```python
from build123d import *

# Parameters (mm, degrees)
F0_W     = 42
F0_H     = 15
F1_DEPTH = 1.5
F2_R     = 3.5
F3_DEPTH = 0.25
F4_R     = 1.25
F5_DEPTH = 5
F6_R     = 1
F7_DEPTH = 5
F9_DEPTH = 1.2


with BuildPart() as f1:
    # F0 (on Top) → F1 (new body)
    with BuildSketch(Plane.XY):
        with Locations((-10.6229138038, 35.7527500853)):
            Rectangle(F0_W, F0_H)
        with BuildLine():
            Line((10.3770861962, 18.2527500853), (10.3770861962, 28.2527500853))
            Line((10.3770861962, 28.2527500853), (-31.6229138038, 28.2527500853))
            Line((-31.6229138038, 28.2527500853), (-31.6229138038, 21.7527500853))
            ThreePointArc((-31.6229138038, 21.7527500853), (-29.8655544909, 17.5101093982), (-25.6229138038, 15.7527500853))
            Line((-25.6229138038, 15.7527500853), (-24.5371273662, 15.7527500853))
            Line((-24.5371273662, 15.7527500853), (-23.1229138038, 15.7527500853))
            Line((-23.1229138038, 15.7527500853), (5.8770861962, 15.7527500853))
            Line((5.8770861962, 15.7527500853), (10.3770861962, 15.7527500853))
            Line((10.3770861962, 15.7527500853), (10.3770861962, 18.2527500853))
        make_face()
        Polygon((43.8770861962, 28.2527500853), (10.3770861962, 28.2527500853), (10.3770861962, 18.2527500853), (31.8770861962, 18.2527500853), (43.8770861962, 18.2527500853), align=None)
        Polygon((31.8770861962, 18.2527500853), (10.3770861962, 18.2527500853), (10.3770861962, 15.7527500853), (22.8770861962, 15.7527500853), (31.8770861962, 15.7527500853), align=None)
        Polygon((22.8770861962, 15.7527500853), (10.3770861962, 15.7527500853), (5.8770861962, 15.7527500853), (5.8770861962, -13.6921136433), align=None)
        Polygon((5.8770861962, -13.6921136433), (5.8770861962, 15.7527500853), (-23.1229138038, 15.7527500853), (-23.1229138038, 11.7527500853), (-23.1229138038, 10.6903063133), (-23.1229138038, -9.6921136433), (-23.1229138038, -13.6921136433), (-2.5732517242, -13.6921136433), (-1.1229138038, -13.6921136433), (2.8770861962, -13.6921136433), (4.2299595661, -13.6921136433), align=None)
        with BuildLine():
            Line((-24.5371273662, 15.7527500853), (-25.6229138038, 15.7527500853))
            add(Edge.make_bspline(
                [(-25.6229138038, 15.7527500853), (-25.2405945212, 15.277672559), (-25.4562471371, 14.5860834187), (-25.3729138038, 14.0027500853)],
                knots=[0, 0, 0, 0, 1.767766953, 1.767766953, 1.767766953, 1.767766953], degree=3))
            ThreePointArc((-25.3729138038, 14.0027500853), (-25.1532438897, 14.9724199994), (-24.5371273662, 15.7527500853))
        make_face()
        with BuildLine():
            Line((-23.1229138038, 11.7527500853), (-23.1229138038, 15.7527500853))
            Line((-23.1229138038, 15.7527500853), (-24.5371273662, 15.7527500853))
            ThreePointArc((-24.5371273662, 15.7527500853), (-25.1532438897, 14.9724199994), (-25.3729138038, 14.0027500853))
            ThreePointArc((-25.3729138038, 14.0027500853), (-24.934409558, 12.6682152852), (-23.7898176859, 11.8538575305))
            ThreePointArc((-23.7898176859, 11.8538575305), (-23.4601761288, 11.7781705466), (-23.1229138038, 11.7527500853))
        make_face()
        with BuildLine():
            Line((-23.1229138038, -13.6921136433), (-23.1229138038, -9.6921136433))
            ThreePointArc((-23.1229138038, -9.6921136433), (-25.1229138038, -11.6921136433), (-23.1229138038, -13.6921136433))
        make_face()
        with BuildLine():
            add(Edge.make_bspline(
                [(2.6500229876, -14.6176919133), (3.1772305838, -14.3094592572), (3.4171862062, -13.6921136433), (4.2299595661, -13.6921136433)],
                knots=[0, 0, 0, 0, 1.8310911299, 1.8310911299, 1.8310911299, 1.8310911299], degree=3))
            Line((4.2299595661, -13.6921136433), (2.8770861962, -13.6921136433))
            ThreePointArc((2.8770861962, -13.6921136433), (2.8194910951, -14.1686251423), (2.6500229876, -14.6176919133))
        make_face()
        with BuildLine():
            ThreePointArc((2.6500229876, -14.6176919133), (2.8194910951, -14.1686251423), (2.8770861962, -13.6921136433))
            Line((2.8770861962, -13.6921136433), (-1.1229138038, -13.6921136433))
            ThreePointArc((-1.1229138038, -13.6921136433), (-1.0673522064, -14.1602581707), (-0.9037545054, -14.6023918402))
            ThreePointArc((-0.9037545054, -14.6023918402), (0.8684756789, -15.692095108), (2.6500229876, -14.6176919133))
        make_face()
        with BuildLine():
            ThreePointArc((-0.9037545054, -14.6023918402), (-1.0673522064, -14.1602581707), (-1.1229138038, -13.6921136433))
            Line((-1.1229138038, -13.6921136433), (-2.5732517242, -13.6921136433))
            add(Edge.make_bspline(
                [(-0.9037545054, -14.6023918402), (-1.4608021595, -14.2992461823), (-1.8808895256, -13.6921136433), (-2.5732517242, -13.6921136433)],
                knots=[0, 0, 0, 0, 1.9015328973, 1.9015328973, 1.9015328973, 1.9015328973], degree=3))
        make_face()
        with BuildLine():
            Line((-23.1229138038, 10.6903063133), (-23.1229138038, 11.7527500853))
            ThreePointArc((-23.1229138038, 11.7527500853), (-23.4601761288, 11.7781705466), (-23.7898176859, 11.8538575305))
            add(Edge.make_bspline(
                [(-23.7898176859, 11.8538575305), (-23.1229138038, 11.3115124404), (-23.3172457665, 11.3592976704), (-23.1229138038, 10.6903063133)],
                knots=[0, 0, 0, 0, 1.3411234928, 1.3411234928, 1.3411234928, 1.3411234928], degree=3))
        make_face()
    extrude(amount=F1_DEPTH)

    # F2 (on face) → F3 (join)
    with BuildSketch(Plane.XY.offset(1.5)):
        with Locations((-20.6229138038, 39.7527500853)):
            Circle(F2_R)
        with Locations((4.3770861962, 37.2527500853)):
            Circle(F2_R)
    extrude(amount=F3_DEPTH)

    # F4 (on face) → F5 (cut)
    with BuildSketch(Plane.XY.offset(1.75)):
        with Locations((4.3770861962, 37.2527500853)):
            Circle(F4_R)
        with Locations((-20.6229138038, 39.7527500853)):
            Circle(F4_R)
    extrude(amount=-F5_DEPTH, mode=Mode.SUBTRACT)

    # F6 (on face) → F7 (cut)
    with BuildSketch(Plane.XY.offset(1.5)):
        with Locations((-28.6229138038, 39.7527500853)):
            Circle(F6_R)
        with Locations((8.3770861962, 32.2527500853)):
            Circle(F6_R)
        with Locations((29.8770861962, 18.2527500853)):
            Circle(F6_R)
        with Locations((-23.1229138038, 14.0027500853)):
            Circle(F6_R)
        with Locations((0.8770861962, -13.6921136433)):
            Circle(F6_R)
    extrude(amount=-F7_DEPTH, mode=Mode.SUBTRACT)

    # F8 (on face) → F9 (join)
    with BuildSketch(Plane.XY.offset(1.5)):
        Polygon((-17.9229138038, -6.7921136433), (-20.4229138038, -6.7921136433), (-20.4229138038, -11.1921136433), (7.3204618692, -11.1921136433), (22.2160988143, 14.6078863567), (-20.4229138038, 14.6078863567), (-20.4229138038, 0.0078863567), (-17.9229138038, 0.0078863567), (-17.9229138038, 1.9078863567), (11.9969990496, 1.9078863567), (5.8770861962, -8.6921136433), (-17.9229138038, -8.6921136433), align=None)
        Polygon((-17.9229138038, 6.0078863567), (-17.9229138038, 12.1078863567), (17.8859717953, 12.1078863567), (14.3641351533, 6.0078863567), align=None, mode=Mode.SUBTRACT)
    extrude(amount=F9_DEPTH)


solid = f1.part
```
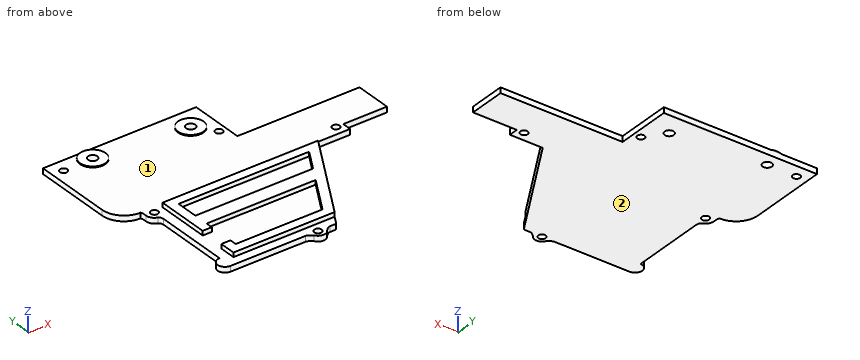
Source: CAD feature listing. Evaluate the final solid. Frame: model axes, mm. Face numbers are marked on the shaded views. Round coordinates to 2 decimals unless told otherwise and drop trailing zeros. Loops run counter-clockwise (first coordinate to the right, second up) from the corner with the lowest first, then second, coordinate; pieces in that order, holes last. Notation, with made-up numbers: M 57,3 L 81,3 A7 ccw 81,7 Z; hole C 5.25,83.5 d11. An arc over 180 degrees is marked long. Use a Markdown table: item, result. Add a question column.
1. Section query C-C on y = 24. Return the cut outline in (x, z), then the cut area to 3 significant figures.
2. Section query D-D on y = 35. Return the cut outline in (x, z), then the cut area to 3 significant figures.
3. Mould query, pull axis Y, two halves, no side actions, for the marked faces 1 and 2. Classes: pulls with the +Y half, pulls with the -Y half, needs draft (parallel to the pull), parting line crosses it, or undercut.
4. Contact query for flat-ended pins moving along their axis: P1, Ø0.8, axis at y = 36, z = 1, coming from the +X side; P2, Ø1.6, axis at x = 30.5, z = 0.5, coming from the +Y side; P3, Ø3, axis at x = 29.88, y = 18.25, coming from the +Z side. Output: stop coordinate, or through.
5. Section query A-A on z = 2.2. Return the cut outline in (x, y).
6. Line query: line 1 (Y direction, x = 1, z = 2.4); line 2 (Y direction, x = -20, z = 1.8); line 3 (Y direction, x = 8.5, z = 1.8). Output: solid intervals per line, ascending.
7. Section query B-B on x = -6. Return the cut outline in (y, z), then the cut area to 3 significant figures.
Reported:
| question | item | result |
|---|---|---|
| 1 | outline | M -31.62,0 L 43.88,0 L 43.88,1.5 L -31.62,1.5 Z |
| 1 | area | 113 mm² |
| 2 | outline | M -31.62,0 L 10.38,0 L 10.38,1.5 L 7.06,1.5 L 7.06,1.75 L 1.7,1.75 L 1.7,1.5 L -31.62,1.5 Z |
| 2 | area | 64.3 mm² |
| 3 | face 1 | undercut |
| 3 | face 2 | needs draft |
| 4 | P1 | stops at x = 10.38 |
| 4 | P2 | stops at y = 28.25 |
| 4 | P3 | stops at z = 1.5 |
| 5 | outline | M -20.42,-11.19 L 7.32,-11.19 L 22.22,14.61 L -20.42,14.61 L -20.42,0.01 L -17.92,0.01 L -17.92,1.91 L 12,1.91 L 5.88,-8.69 L -17.92,-8.69 L -17.92,-6.79 L -20.42,-6.79 Z; hole M -17.92,6.01 L 14.36,6.01 L 17.89,12.11 L -17.92,12.11 Z |
| 6 | line 1 | y = -11.19 to -8.69, 1.91 to 6.01, 12.11 to 14.61 |
| 6 | line 2 | y = -11.19 to -6.79, 0.01 to 14.61 |
| 6 | line 3 | y = -9.15 to -4.15, 1.91 to 6.01, 12.11 to 14.61 |
| 7 | outline | M -13.69,0 L 43.25,0 L 43.25,1.5 L 14.61,1.5 L 14.61,2.7 L 12.11,2.7 L 12.11,1.5 L 6.01,1.5 L 6.01,2.7 L 1.91,2.7 L 1.91,1.5 L -8.69,1.5 L -8.69,2.7 L -11.19,2.7 L -11.19,1.5 L -13.69,1.5 Z |
| 7 | area | 96.3 mm² |
